Geometry: final body of the model. Coordinates: model frame, mm. Face numbers are marked on the shaded views. A direction names the side the tool comes from. Give positions to 0.01 mm unless a question says otherwise; leave off trailing zeros. Write each loop counter-clockwise with the first axis right and the second up, starting at its lowest first coordinate (ties: lowest second). Pieces come first, ordered by that corner, then holes. Notation, with made-up numbers: (7, 48) -> (59, 48) arc R19 cw to (59, 82) -> close; hole circle Ø2 at (-1.75, 12.25). An arc over 180 degrees is marked (long way). Answer in a Markdown table with one row per item. Add a question column.
Item 1: Section query B-B on y = 0.25. Output: boundary loops of the cut face in (x, z).
Item 2: Section query D-D on z = -3.25. Output: boundary loops of the cut face in (x, y).
Item 3: Material intervals for probe 1 along Y at (x, z) = (-1.75, -3.75); probe 2 along Y at (x, z) = (2.25, 0); probe 3 along X at (y, z) = (4.8, 0), sorted ascending. Write a range as from..to.
Item 4: Draft query along Y for the marked faces 1, 2 and 3. Return one class per face: +Y half, -Y half, draft (parallel to the pull), parting line (faces both ways), or undercut.
Item 5: First-contact query: P1, Ø0.6, axis at x = -1.5, y = 3, coming from the +Z side; P2, Ø2, axis at y = 1, z = 3, coming from the +X side; P3, Ø1.1, axis at y = -0.5, z = -5, coming from the +X side; P4, Ø2, axis at x = 0, z = 0, coming from the +Y side. Flat tips, straight axial feed; report the tip coordinate or a pass-through.
Item 6: Section query C-C on y = 3.25. Output: boundary loops of the cut face in (x, z).
Item 7: Access query for the marked faces 4, 5 and 6. Directions: +Z, -Z, +X, -X, +Y, -Y. A direction counts if a zero-diameter tool reaches every point of the face in a straight line with its end or side. Return the directions, or none.
Item 8: Section query A-A on x = 2.5. Output: boundary loops of the cut face in (y, z).
Autodesk Inventor part; units mm, degrees
ref_plane "YZ Plane" through (0, 0, 0) normal (1, 0, 0) x (0, 1, 0)
ref_plane "XZ Plane" through (0, 0, 0) normal (0, 1, 0) x (-1, 0, 0)
ref_plane "XY Plane" through (0, 0, 0) normal (0, 0, 1) x (1, 0, 0)
sketch "スケッチ1" plane through (0, 0, 0) normal (0, 1, 0) x (-1, 0, 0)
  circle A0 centre (0, 0) radius 1.15
  circle A1 centre (0, 0) radius 2
  circle A2 centre (0, 0) radius 3.5
  line L0 (0, 0) -> (0, 3.5)
  line L1 (2, 0) -> (-2, 0)
  line L2 (2, 0) -> (2, -2.8723)
  line L3 (-2, 0) -> (-2, -2.8723)
  line L4 (0, 2) -> (3.5, 2)
  line L5 (3.5, 2) -> (3.5, 6)
  line L6 (3.5, 6) -> (0, 6)
  line L7 (0, 6) -> (0, 2)
  line L8 (0, 6) -> (3.5, 6)
  line L9 (3.5, 6) -> (3.5, 0)
  line L10 (3.5, 0) -> (0, 0)
  line L11 (0, 0) -> (0, 6)
  line L12 (0, 0) -> (0, -8)
  line L13 (0, 0) -> (3.5, 0)
  line L14 (3.5, 0) -> (3.5, -8)
  line L15 (3.5, -8) -> (0, -8)
  line L16 (0, -8) -> (0, 0)
  line L17 (2, -2.8723) -> (2, -8)
  line L18 (0, -8) -> (3.5, -4.5)
  line L19 (0, -8) -> (4.9497, -8) construction
  point P0 (2, -6)
  point P1 (0, -3.5)
  dimension "d0" = 2.3
  dimension "d1" = 4
  dimension "d2" = 7
  dimension "d3" = 3.5
  dimension "d4" = 4
  dimension "d5" = 8
  dimension "d6" = 45
extrude "押し出し1" add sketch "スケッチ1" along normal blind 3 contours A1 L3 A2 L0
extrude "押し出し2" add sketch "スケッチ1" along normal blind 4.5 contours L10 A2 L2 | A1 L4 A2 L10 | L0 A2 L4 | A2 L14 L18 L17 | A2 L4 L9 | L7 L6 L5 L4 A2
extrude "押し出し3" add sketch "スケッチ1" against normal blind 1 contours L1 A1 L12 A0 | A0 L0 A1 L1 | A0 L1 A1 L0 | L12 A1 L1 A0 | L2 A2 L12 A1 | L10 A2 L2 | A1 L4 A2 L10 | A1 L3 A2 L0 | L0 A2 L4 | L12 A2 L3 A1 | L17 L18 L12 A2 | A2 L14 L18 L17 | A2 L4 L9 | L7 L6 L5 L4 A2
sketch "スケッチ2" plane through (0, 4.5, 0) normal (0, 1, 0) x (1, 0, 0)
  circle A0 centre (0, 0) radius 1.15
  circle A1 centre (0, 0) radius 2
  circle A2 centre (0, 0) radius 3.5
  line L0 (0, -2) -> (0, -3.5)
  line L1 (-3.5, 4.5) -> (-3.5, -6)
  line L2 (0, -2) -> (-3.5, -2)
  line L3 (-3.5, -2) -> (-3.5, -6)
  line L4 (-3.5, -6) -> (0, -6)
  line L5 (0, -6) -> (0, -2)
  line L6 (0, -2) -> (-3.5, -2)
  line L7 (-3.5, -2) -> (-3.5, 8)
  line L8 (-3.5, 8) -> (0, 8)
  line L9 (0, 8) -> (0, -2)
  line L10 (0, 0) -> (-2, 0)
  line L11 (-2, 0) -> (-2, 8)
  line L12 (-2, 8) -> (0, 8)
  line L13 (0, 8) -> (0, 0)
  line L14 (0, 8) -> (-3.5, 4.5)
  line L15 (0, 8) -> (4.9497, 8) construction
  point P0 (0, 3.5)
  dimension "d14" = 4
  dimension "d15" = 7
  dimension "d13" = 2.3
  dimension "d16" = 3.5
  dimension "d17" = 4
  dimension "d18" = 3.5
  dimension "d19" = 10
  dimension "d20" = 2
  dimension "d21" = 8
  dimension "d22" = 135
extrude "押し出し4" add sketch "スケッチ2" along normal blind 1 contours A0 L9 A1 | A0 L10 A1 L9 | L9 A1 L10 A0 | L9 A2 L0 A1 | A1 L11 A2 L9 | L2 A2 L11 A1 | L0 A2 L2 | A2 L11 L14 L9 | L5 L4 L1 L2 A2 | L2 L1 A2 | A2 L1 L14 L11
sketch "スケッチ3" plane through (-3.5, -1, 6) normal (0, 0, 1) x (1, 0, 0)
  line L0 (0, 0) -> (0, 6.5)
  line L1 (0, 0) -> (3.5, 0)
  line L2 (3.5, 0) -> (3.5, 1)
  line L3 (3.5, 1) -> (0, 1)
  line L4 (0, 1) -> (0, 0)
  line L5 (3.5, 1) -> (2, 1)
  line L6 (2, 1) -> (2, 1.5)
  line L7 (2, 1.5) -> (3.5, 1.5)
  line L8 (3.5, 1.5) -> (3.5, 1)
  circle A0 centre (2, 1.5) radius 0.5
  line L9 (0, 6.5) -> (1.75, 6.5)
  line L10 (1.75, 6.5) -> (1.75, 4.25)
  line L11 (1.75, 4.25) -> (0, 4.25)
  line L12 (0, 4.25) -> (0, 6.5)
  dimension "d25" = 3.5
  dimension "d26" = 1
  dimension "d27" = 1.5
  dimension "d28" = 0.5
  dimension "d29" = 1.75
  dimension "d30" = 2.25
extrude "押し出し5" cut sketch "スケッチ3" against normal blind 6 contours A0 L7 L6 | L6 L7 A0
hole "穴1" at (-1.75, 3.25, 6) direction (0, 0, -1) diameter 2.1 depth 4
properties part number "rod6.0"
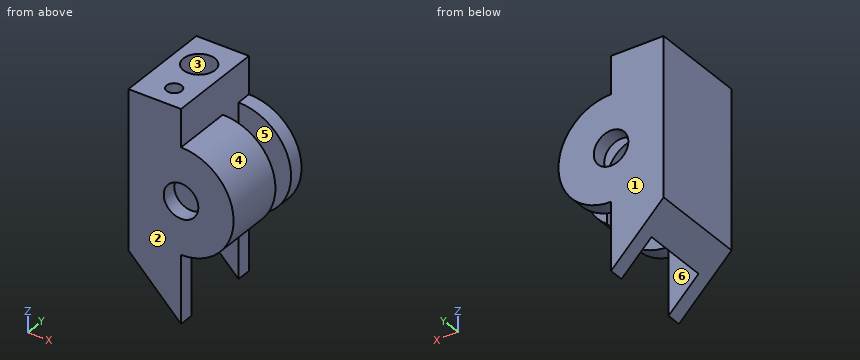
Findings below:
| question | item | result |
|---|---|---|
| 1 | outline | (-3.5, -4.5) -> (-2, -6) -> (-2, 0) arc R2 cw to (-1.93, 0.51) -> (-1.93, 6) -> (-3.5, 6) -> close; (-1.07, 1.69) arc R2 cw to (2, 0) -> (2, -2.87) arc R3.5 ccw to (0, 3.5) -> (0, 6) -> (-1.07, 6) -> close |
| 2 | outline | (-3.5, -1) -> (1.3, -1) -> (1.3, 0) -> (-2, 0) -> (-2, 4.5) -> (1.3, 4.5) -> (1.3, 5.5) -> (-3.5, 5.5) -> close |
| 3 | probe 1 | y = -1..0, 4.5..5.5 |
| 3 | probe 2 | y = -1..3, 4.5..5.5 |
| 3 | probe 3 | x = -3.5..-1.15, 1.15..3.5 |
| 4 | face 1 | +Y half |
| 4 | face 2 | -Y half |
| 4 | face 3 | undercut |
| 5 | P1 | stops at z = 2 |
| 5 | P2 | stops at x = 2.87 |
| 5 | P3 | stops at x = 0 |
| 5 | P4 | passes through |
| 6 | outline | (-3.5, -4.5) -> (-2, -6) -> (-2, 0) arc R2 cw to (0, 2) -> (0, 6) -> (-0.7, 6) -> (-0.7, 2) -> (-2.8, 2) -> (-2.8, 6) -> (-3.5, 6) -> close |
| 7 | face 4 | +X, +Y, -Y |
| 7 | face 5 | -Z, +X |
| 7 | face 6 | -Z |
| 8 | outline | (-1, -2.45) -> (3, -2.45) -> (3, 2.45) -> (-1, 2.45) -> close; (4.5, -2.45) -> (5.5, -2.45) -> (5.5, 2.45) -> (4.5, 2.45) -> close |
